For this review, take the finished solid that the model builds, in its own axes (mm). Face numbers are marked on the shaded views. Round coordinates to 2 decimals unless told otherwise and drop trailing zeros. Order: outer loops, then holes, each group sorted by start corner. A loop starts at its lowest first (then second) coordinate and runs counter-clockwise, first axis right, second up. Notation, with made-up numbers: (-17.5, 26.5) -> (2.5, 26.5) arc R17 ccw to (2.5, 30.5) -> close; hole circle Ø10 at (74, 83.25). An arc over 180 degrees is marked (long way). Answer in a Markdown table with one row per item.
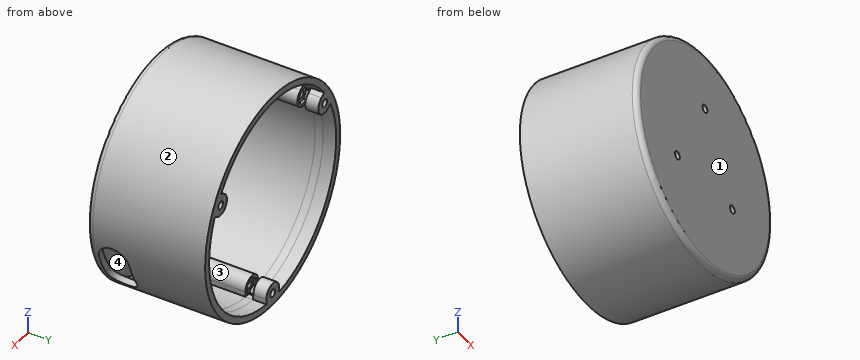
```python
from build123d import *

# Parameters (mm, degrees)
SKETCH1_R           = 42.5
BOSS_EXTRUDE1_DEPTH = 45
FILLET1_R           = 2
SHELL1_T            = -2.5
SKETCH2_R           = 1.5
BOSS_EXTRUDE2_DEPTH = 42.5
CUT_EXTRUDE1_START  = -3
CUT_EXTRUDE1_DEPTH  = 6
CUT_EXTRUDE2_START  = -5
SKETCH4_R           = 40
CUT_EXTRUDE2_DEPTH  = 3
CUT_EXTRUDE3_DEPTH  = 120
SKETCH7_R           = 1.5
CUT_EXTRUDE4_DEPTH  = 10


with BuildPart() as part:
    # Sketch1 → Boss-Extrude1 (new body)
    with BuildSketch(Plane(origin=(0, 0, 0), x_dir=(1, 0, 0), z_dir=(0, 1, 0))):
        with Locations(Location((0, 0, 0), (0, 0, 90))):
            Circle(SKETCH1_R)
    extrude(amount=BOSS_EXTRUDE1_DEPTH)

    # Fillet1
    fillet1_edges = [part.edges().sort_by_distance(p)[0] for p in [
        (0, 0, 42.5),
    ]]
    fillet(fillet1_edges, radius=FILLET1_R)

    # Shell1
    shell1_openings = [part.faces().sort_by_distance(p)[0] for p in [
        (0, 45, 0),
    ]]
    offset(amount=SHELL1_T, openings=shell1_openings, kind=Kind.INTERSECTION)

    # Sketch2 → Boss-Extrude2 (add)
    with BuildSketch(Plane(origin=(0, 2.5, 0), x_dir=(1, 0, 0), z_dir=(0, 1, 0))):
        with BuildLine():
            Line((-34.080943597, -24.295444113), (-30.735760263, -22.364101615))
            ThreePointArc((-30.735760263, -22.364101615), (-29.271658648, -16.9), (-34.735760263, -15.435898385))
            Line((-34.735760263, -15.435898385), (-38.080943597, -17.367240883))
            Line((-38.080943597, -17.367240883), (-34.080943597, -24.295444113))
        make_face()
        with Locations(Location((-32.735760263, -18.9, 0), (0, 0, 90))):
            Circle(SKETCH2_R, mode=Mode.SUBTRACT)
        with BuildLine():
            Line((38.080943597, -17.367240883), (34.735760263, -15.435898385))
            ThreePointArc((34.735760263, -15.435898385), (29.271658648, -16.9), (30.735760263, -22.364101615))
            Line((30.735760263, -22.364101615), (34.080943597, -24.295444113))
            Line((34.080943597, -24.295444113), (38.080943597, -17.367240883))
        make_face()
        with Locations(Location((32.735760263, -18.9, 0), (0, 0, 90))):
            Circle(SKETCH2_R, mode=Mode.SUBTRACT)
        with BuildLine():
            Line((-4, 41.662684996), (-4, 37.8))
            ThreePointArc((-4, 37.8), (0, 33.8), (4, 37.8))
            Line((4, 37.8), (4, 41.662684996))
            Line((4, 41.662684996), (-4, 41.662684996))
        make_face()
        with Locations(Location((0, 37.8, 0), (0, 0, 90))):
            Circle(SKETCH2_R, mode=Mode.SUBTRACT)
    extrude(amount=BOSS_EXTRUDE2_DEPTH)

    # Sketch3 → Cut-Extrude1 (cut)
    with BuildSketch(Plane(origin=(0, 45, 0), x_dir=(1, 0, 0), z_dir=(0, 1, 0)).offset(CUT_EXTRUDE1_START)):
        Polygon((-31.119179509, -16.1), (-34.352341017, -16.1), (-35.968921771, -18.9), (-34.352341017, -21.7), (-31.119179509, -21.7), (-29.502598756, -18.9), align=None)
        Polygon((0, 41.033161507), (-2.8, 39.416580754), (-2.8, 36.183419246), (0, 34.566838493), (2.8, 36.183419246), (2.8, 39.416580754), align=None)
        Polygon((34.352341017, -16.1), (31.119179509, -16.1), (29.502598756, -18.9), (31.119179509, -21.7), (34.352341017, -21.7), (35.968921771, -18.9), align=None)
    extrude(amount=-CUT_EXTRUDE1_DEPTH, mode=Mode.SUBTRACT)

    # Sketch4 → Cut-Extrude2 (cut)
    with BuildSketch(Plane(origin=(0, 45, 0), x_dir=(1, 0, 0), z_dir=(0, 1, 0)).offset(CUT_EXTRUDE2_START)):
        Circle(SKETCH4_R)
    extrude(amount=-CUT_EXTRUDE2_DEPTH, mode=Mode.SUBTRACT)

    # Sketch6 → Cut-Extrude3 (cut)
    with BuildSketch(Plane(origin=(0, 0, 0), x_dir=(0, 0, -1), z_dir=(1, 0, 0))):
        with BuildLine():
            Line((12.858520148, 14.864349815), (22.241479852, 14.864349815))
            ThreePointArc((22.241479852, 14.864349815), (28.105829667, 9), (22.241479852, 3.135650185))
            Line((22.241479852, 3.135650185), (12.858520148, 3.135650185))
            ThreePointArc((12.858520148, 3.135650185), (6.994170333, 9), (12.858520148, 14.864349815))
        make_face()
    extrude(amount=CUT_EXTRUDE3_DEPTH, mode=Mode.SUBTRACT)

    # Sketch7 → Cut-Extrude4 (cut)
    with BuildSketch(Plane.XZ):
        with Locations(Location((17.320508076, -10, 0), (0, 0, 270))):
            Circle(SKETCH7_R)
        with Locations(Location((0, 20, 0), (0, 0, 270))):
            Circle(SKETCH7_R)
        with Locations(Location((-17.320508076, -10, 0), (0, 0, 270))):
            Circle(SKETCH7_R)
    extrude(amount=-CUT_EXTRUDE4_DEPTH, mode=Mode.SUBTRACT)


solid = part.part
```
Q1. The part is to be moulded in two halves that separate along Z. For the marked faces 1, 2, 3 and 4, say which applies: +Z half, -Z half, draft (parallel to the pull), parting line (faces both ways), or undercut.
Answer key:
| item | result |
|---|---|
| face 1 | draft |
| face 2 | parting line |
| face 3 | undercut |
| face 4 | undercut |
Q2. Take a section at A-A, the plane y = 18.5. Write out the cut boundary in (x, z).
Answer key:
| item | result |
|---|---|
| outline | circle Ø85 at (0, 0); hole (-36.47, 16.44) arc R40 ccw to (-4, -39.8) -> (-4, -37.8) arc R4 cw to (4, -37.8) -> (4, -39.8) arc R40 ccw to (36.47, 16.44) -> (34.74, 15.44) arc R4 cw to (30.74, 22.36) -> (32.47, 23.36) arc R40 ccw to (-32.47, 23.36) -> (-30.74, 22.36) arc R4 cw to (-34.74, 15.44) -> close; hole circle Ø3 at (-32.74, 18.9); hole circle Ø3 at (0, -37.8); hole circle Ø3 at (32.74, 18.9) |
Q3. Clearance check with flat-ended pins moving along their axes: pin 1 Ø0.9 at (x, z) = (-32, 19.5) entering from +Y; pin 2 Ø12 at (y, z) = (35.5, -31) entering from -X; pin 3 Ø4 at (x, z) = (-33, 18) entering from +Y; pin 4 Ø0.8 at (x, y) = (33, 36.5) entering from +Z. State where each tip first meets the part, or that it passes through.
Answer key:
| item | result |
|---|---|
| pin 1 | stops at y = 2.5 |
| pin 2 | stops at x = -34.37 |
| pin 3 | stops at y = 45 |
| pin 4 | stops at z = 27.27 |
Q4. To check wall thickness, follow probe 1 along X at (y, z) = (23.5, 18.9); probe 2 along X at (y, z) = (5, 0.5); probe 3 along Y at (x, z) = (-30.5, -19.5). State the ranges of each line that lie inside material, in increasing order.
Answer key:
| item | result |
|---|---|
| probe 1 | x = -38.07 to -34.24, -31.24 to -28.74, 28.74 to 31.24, 34.24 to 38.07 |
| probe 2 | x = -42.5 to -40, 40 to 42.5 |
| probe 3 | y = 0 to 2.5 |
Q5. Take a section at B-B, the plane y = 9. Write out the cut boundary in (x, z), then the cut area to 3 significant figures.
Answer key:
| item | result |
|---|---|
| outline | (-36.47, 16.44) -> (-34.74, 15.44) arc R4 ccw to (-30.74, 22.36) -> (-32.47, 23.36) arc R40 cw to (32.47, 23.36) -> (30.74, 22.36) arc R4 ccw to (34.74, 15.44) -> (36.47, 16.44) arc R40 cw to (39.38, -6.99) -> (41.92, -6.99) arc R42.5 ccw (long way) to (31.88, -28.11) -> (28.46, -28.11) arc R40 cw to (4, -39.8) -> (4, -37.8) arc R4 ccw to (-4, -37.8) -> (-4, -39.8) arc R40 cw to start; hole circle Ø3 at (-32.74, 18.9); hole circle Ø3 at (0, -37.8); hole circle Ø3 at (32.74, 18.9) |
| area | 694 mm^2 |
